from build123d import *

# Parameters (mm, degrees)
BOSS_EXTRUDE1_DEPTH      = 20
BOSS_EXTRUDE1_DEPTH_BACK = 1
SKETCH1_R                = 75
FILLET1_R                = 5
BOSS_EXTRUDE2_DEPTH      = 5
CHAMFER1_SIZE            = 2.5
FILLET2_R                = 5
SKETCH4_R                = 10
BOSS_EXTRUDE3_DEPTH      = 5
CHAMFER2_SIZE            = 2.5
SKETCH5_R                = 5
CUT_EXTRUDE1_DEPTH       = 10


with BuildPart() as part:
    # Sketch1 → Boss-Extrude1 (new, two sides: drawn at the far end of the back side and taken through both)
    with BuildSketch(Plane(origin=(0, 0, 0), x_dir=(1, 0, 0), z_dir=(0, 1, 0)).offset(-BOSS_EXTRUDE1_DEPTH_BACK)):
        with Locations(Location((0, 0, 0), (0, 0, 270))):
            Circle(SKETCH1_R)
    extrude(amount=BOSS_EXTRUDE1_DEPTH + BOSS_EXTRUDE1_DEPTH_BACK)

    # Fillet1
    fillet1_edges = [part.edges().sort_by_distance(p)[0] for p in [
        (0, 20, -75),
    ]]
    fillet(fillet1_edges, radius=FILLET1_R)

    # Sketch3 → Boss-Extrude2 (add, symmetric)
    with BuildSketch(Plane.XY):
        with BuildLine():
            Line((-35, 15), (30, 15))
            ThreePointArc((30, 15), (17.428098582, 56.126843631), (14.970645506, 99.06203778))
            ThreePointArc((14.970645506, 99.06203778), (6.012327577, 113.742340307), (-10.849201429, 110.358321696))
            ThreePointArc((-10.849201429, 110.358321696), (-35.460543036, 65.854059614), (-35, 15))
        make_face()
    extrude(amount=BOSS_EXTRUDE2_DEPTH, both=True)

    # Chamfer1
    chamfer1_edges = [part.edges().sort_by_distance(p)[0] for p in [
        (-34.796467261, 68.341174934, -5),
        (16.970295051, 58.803839559, -5),
        (6.012327577, 113.742340307, -5),
        (16.970295051, 58.803839559, 5),
        (6.012327577, 113.742340307, 5),
        (-34.796467261, 68.341174934, 5),
    ]]
    chamfer(chamfer1_edges, length=CHAMFER1_SIZE)

    # Fillet2
    fillet2_edges = [part.edges().sort_by_distance(p)[0] for p in [
        (-4.241511046, 20, -5),
        (-4.241511046, 20, 5),
    ]]
    fillet(fillet2_edges, radius=FILLET2_R)

    # Sketch4 → Boss-Extrude3 (add)
    with BuildSketch(Plane.XY.offset(5)):
        with Locations(Location((0, 100, 0), (0, 0, 180))):
            Circle(SKETCH4_R)
    extrude(amount=BOSS_EXTRUDE3_DEPTH)

    # Chamfer2
    chamfer2_edges = [part.edges().sort_by_distance(p)[0] for p in [
        (10, 100, 10),
    ]]
    chamfer(chamfer2_edges, length=CHAMFER2_SIZE)

    # Sketch5 → Cut-Extrude1 (cut)
    with BuildSketch(Plane(origin=(0, 0, -5), x_dir=(-1, 0, 0), z_dir=(0, 0, -1))):
        with Locations((0, 100)):
            Circle(SKETCH5_R)
    extrude(amount=-CUT_EXTRUDE1_DEPTH, mode=Mode.SUBTRACT)


solid = part.part
Input: part model. Units: mm. Frame: model coordinates. A direction names the side the tool comes from. Give positions to 0.01 mm unless a question says otherwise; leave off trailing zeros. Write each loop counter-clockwise with the first axis right and the second up, starting at its lowest first coordinate (ties: lowest second). Pieces come first, ordered by that corner, then holes. Notation, with made-up numbers: M -38,21 L 8,21 A21 cw 8,57 Z; hole C 19,46 d10. An arc over 180 degrees is marked long. Write item = value, one per line. Start each with the question number.
1) First-contact query: pin 1 Ø4.5 at (x, y) = (-3, 103.5) entering from +Z; pin 2 Ø4 at (x, y) = (-54.5, 13) entering from +Z; pin 3 Ø2 at (x, z) = (38.5, -46) entering from +Y. Flat tips, straight axial feed; report the tip coordinate or a pass-through.
2) Cut plane A-A on z = 0. Return the cut outline in (x, y).
3) Draft query along Y for faces 4 (the flat face through (1, -1, -1)), 5 (the flat face through (0, 100, 10)), 6 (the cylindrical face through (-5, 21, 7)), 7 (the cylindrical face through (1.302, 90.085, 6.232)). Return one class per face: +Y half, -Y half, draft (parallel to the pull), parting line (faces both ways), or undercut.
4) Cut plane B-B on x = 0. Return the cut outline in (y, z), then the cut area to 3 significant figures.
5) Cut plane C-C on y = 7.5. Return the cut outline in (x, z).
6) Reachability of faces 1 (the cylindrical face through (1.08, 95.12, -0.07)), 2 (the flat face through (-7, 60, -5)), 3 (the cylindrical face through (17.06, 58.25, 0.04)) from +Z, -Z, +X, -X, +Y, -Y: full face, straight path, thin tool, end or side. Return the list, or none.
7) Material intervals for line 1 along Y through (x, z) = (0, -1.5); line 2 along Y through (x, z) = (-28, 44); line 3 along Z through (x, y) = (-1.5, 105), sorted ascending. Write a range as [from, to].
Solved:
q1.pin_1 = 10
q1.pin_2 = 53.56
q1.pin_3 = 20
q2.outline = M -75,-1 L 75,-1 L 75,15 A5 ccw 70,20 L 27.88,20 A180 cw 14.97,99.06 A15 ccw -10.85,110.36 A100 ccw -36.23,20 L -70,20 A5 ccw -75,15 Z; hole C 0,100 d10
q3.face_4 = -Y half
q3.face_5 = draft
q3.face_6 = undercut
q3.face_7 = undercut
q4.outline = M -1,-75 L 15,-75 A5 ccw 20,-70 L 20,-10 A5 cw 25,-5 L 95,-5 L 95,5 L 105,5 L 105,-5 L 112.5,-5 L 115,-2.5 L 115,2.5 L 112.5,5 L 110,5 L 110,7.5 L 107.5,10 L 92.5,10 L 90,7.5 L 90,5 L 25,5 A5 cw 20,10 L 20,70 A5 ccw 15,75 L -1,75 Z
q4.area = 4,090 mm2
q5.outline = C 0,0 d150
q6.face_1 = -Z
q6.face_2 = -Z, +X, -X, +Y
q6.face_3 = +Z, -Z, +X
q7.line_1 = [-1, 95], [105, 115]
q7.line_2 = [-1, 20]
q7.line_3 = [-5, 10]
